Here's how the part is built. I have some questions about the finished solid (model axes, mm). Face numbers are marked on the shaded views. Round coordinates to 2 decimals unless told otherwise and drop trailing zeros. Write each loop counter-clockwise with the first axis right and the second up, starting at its lowest first coordinate (ties: lowest second). Pieces come first, ordered by that corner, then holes. Notation, with made-up numbers: M 66,64 L 78,64 A10 cw 78,69 Z; hole C -33,20.5 d4. An arc over 180 degrees is marked long. Use one line per item in the form item = value. Start each with the question number.
Q1. I'm going to push flat-ended pins straight in: pin 1 Ø1.5 at (x, z) = (-9, 30.5) entering from -Y; pin 2 Ø1 at (y, z) = (0.5, 32) entering from +X; pin 3 Ø2 at (y, z) = (-0.5, 22.5) entering from +X; pin 4 Ø10 at (x, y) = (10, 2.5) entering from +Z. Where does each tip first touch, or does it pass through?
Q2. We'd pull the mould along Z, two halves only. Please class the marked faces 1, 2 and 3: +Z half, -Z half, draft (parallel to the pull), parting line (faces both ways), or undercut.
Q3. I want a section at A-A on x = 0. List the corners of the cut face in (y, z) for me.
Q4. I need wall thicknesses on line 1 along X through (y, z) = (1, 20.5); line 2 along X through (y, z) = (2.5, 25.5); line 3 along Y through (x, z) = (4, 38). Which ranges of each line are inside material? Lowest first, please. Write a range as from..to.
Q5. I want a section at B-B on z = 12. List the corners of the cut face in (x, y) for me, and give its area (3 significant figures).
Q6. I want a section at C-C on z = 3. List the corners of the cut face in (x, y) for me, and give its area (3 significant figures).
```python
from build123d import *

# Parameters (mm, degrees)
F0_R      = 14.5
F2_R      = 15.25
F3_FACE_R = 15.25
F5_R      = 13
F6_FACE_R = 13
F8_R      = 14.5
F10_T     = -2


with BuildPart() as f3:
    # F0 (on Top) → F3 section 0
    with BuildSketch(Plane.XY):
        Circle(F0_R)
    # F2 (on offset) → F3 section 1
    with BuildSketch(Plane.XY.offset(5)):
        Circle(F2_R)
    loft()

    # F3_face (on face) → F6 section 0
    with BuildSketch(Plane.XY.offset(5)):
        Circle(F3_FACE_R)
    # F5 (on offset) → F6 section 1
    with BuildSketch(Plane.XY.offset(30)):
        Circle(F5_R)
    loft()

    # F6_face (on face) → F9 section 0
    with BuildSketch(Plane.XY.offset(30)):
        Circle(F6_FACE_R)
    # F8 (on offset) → F9 section 1
    with BuildSketch(Plane.XY.offset(40)):
        Circle(F8_R)
    loft()

    # F10
    f10_openings = [f3.faces().sort_by_distance(p)[0] for p in [
        (0, 0, 40),
        (0, 0, 0),
    ]]
    offset(amount=F10_T, openings=f10_openings, kind=Kind.INTERSECTION)


solid = f3.part
```
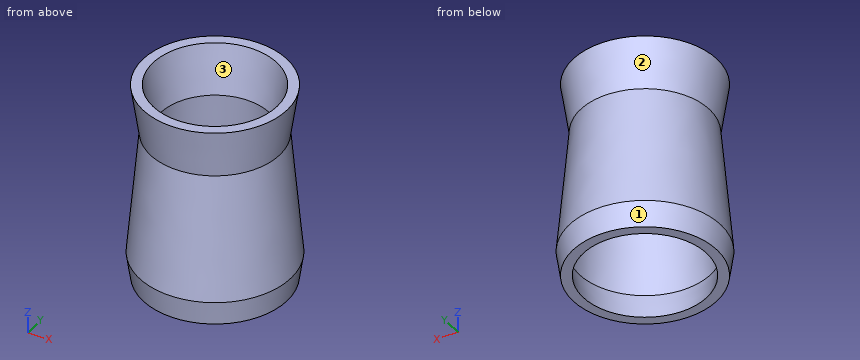
Reported:
q1.pin_1 = -10.16
q1.pin_2 = 13.37
q1.pin_3 = 13.76
q1.pin_4 = 40
q2.face_1 = -Z half
q2.face_2 = undercut
q2.face_3 = +Z half
q3.outline = M -15.25,5 L -14.5,0 L -12.48,0 L -13.24,5.06 L -10.99,30.06 L -12.48,40 L -14.5,40 L -13,30 Z; M 10.99,30.06 L 13.24,5.06 L 12.48,0 L 14.5,0 L 15.25,5 L 13,30 L 14.5,40 L 12.48,40 Z
q4.line_1 = -13.82..-11.8, 11.8..13.82
q4.line_2 = -13.17..-11.12, 11.12..13.17
q4.line_3 = -13.62..-11.5, 11.5..13.62
q5.outline = C 0,0 d29.24; hole C 0,0 d25.22
q5.area = 172 mm^2
q6.outline = C 0,0 d29.9; hole C 0,0 d25.86
q6.area = 177 mm^2
